from build123d import *

# Parameters (mm, degrees)
F2_DEPTH = 5
F1_W     = 60
F1_H     = 60
F3_DEPTH = 2


# Not quite as in the source:
# - ends of sketch curves that miss each other by under 0.0002 mm in the source are joined


with BuildPart() as f2:
    # F0 (on Top) → F2 (new body)
    with BuildSketch(Plane.XY):
        with BuildLine():
            Line((12.5301, 15.3483), (13.2754, 18.8292))
            ThreePointArc((13.2754, 18.8292), (-0.0620714554, 21.313337159), (-13.4587020592, 19.1710971727))
            Line((-13.4587020592, 19.1710971727), (-12.8601, 15.6049))
            Line((-12.8601, 15.6049), (-0.5682, 9.3636))
            Line((-0.5682, 9.3636), (12.5301, 15.3483))
        make_face()
        Polygon((5.0768, 17.1559), (-0.2261, 13.5284), (-5.468, 17.1559), align=None, mode=Mode.SUBTRACT)
    extrude(amount=F2_DEPTH)



with BuildPart() as f2b:
    # F0 (on Top) → F2, piece 2 (new body)
    with BuildSketch(Plane.XY):
        Polygon((20.3255, 19.4397), (14.8884, 19.4397), (13.6053, 14.2734), (4.869, 10.0354), (3.3296, 1.7791), (12.2, 1.7791), (17.6374, 5.1989), align=None)
        Polygon((15.3523, 8.6188), (15.3523, 7.3484), (5.7369, 3.3912), (5.7369, 4.9303), align=None, mode=Mode.SUBTRACT)
        Polygon((16.3548, 12.6613), (16.3548, 11.2445), (6.9587, 7.5562), (6.9587, 8.9606), align=None, mode=Mode.SUBTRACT)
    extrude(amount=F2_DEPTH)


with BuildPart() as f2c:
    # F0 (on Top) → F2, piece 3 (new body)
    with BuildSketch(Plane.XY):
        Polygon((-4.0627, 1.9012), (-5.6145, 10.2308), (-13.9352, 14.5301), (-15.0105, 19.9041), (-20.3255, 19.9041), (-17.8452, 5.7363), (-12.3223, 1.9012), align=None)
        Polygon((-16.098, 9.4248), (-6.3597, 5.3332), (-6.3597, 3.9288), (-15.9514, 8.1913), align=None, mode=Mode.SUBTRACT)
        Polygon((-16.6601, 13.6628), (-7.2887, 9.4248), (-7.2152, 7.947), (-16.5379, 12.1483), align=None, mode=Mode.SUBTRACT)
    extrude(amount=F2_DEPTH)


with BuildPart() as f2d:
    # F0 (on Top) → F2, piece 4 (new body)
    with BuildSketch(Plane.XY):
        Polygon((-14.0697, -1.5185), (-14.4852, 1.7669), (-17.5644, 3.7209), (-16.3667, -15.1486), (-9.0357, -18.9712), (-8.9623, -4.7428), align=None)
    extrude(amount=F2_DEPTH)


with BuildPart() as f2e:
    # F0 (on Top) → F2, piece 5 (new body)
    with BuildSketch(Plane.XY):
        Polygon((17.161, 3.318), (13.6663, 0.8999), (13.5321, -1.6531), (8.0952, -4.938), (8.0952, -19.2404), (15.6947, -15.8937), align=None)
    extrude(amount=F2_DEPTH)


with BuildPart() as f2f:
    # F0 (on Top) → F2, piece 6 (new body)
    with BuildSketch(Plane.XY):
        Polygon((-3.794, 9.2295), (-2.6575, 2.3167), (-2.6575, -10.5809), (1.8513, -10.5809), (1.8513, 2.4509), (3.1219, 9.2295), (-0.5682, 7.6783), align=None)
    extrude(amount=F2_DEPTH)


with BuildPart() as f2g:
    # F0 (on Top) → F2, piece 7 (new body)
    with BuildSketch(Plane.XY):
        Polygon((-7.4959, -4.7428), (-7.4959, -19.4476), (-6.0788, -20.4494), (-4.1971, -14.2084), (3.1219, -14.2084), (5.0647, -20.3757), (6.6777, -19.5086), (6.6777, -4.7428), (3.3906, -1.7137), (3.3906, -11.8511), (-4.0627, -11.8511), (-4.1971, -1.7137), align=None)
    extrude(amount=F2_DEPTH)


with BuildPart() as f2h:
    # F0 (on Top) → F2, piece 8 (new body)
    with BuildSketch(Plane.XY):
        Polygon((-3.2564, -15.5518), (-4.7349, -21.3286), (3.7325, -21.3286), (2.047, -15.5518), align=None)
    extrude(amount=F2_DEPTH)


with BuildPart() as f2_1:
    add(f2.part)

    add(f2b.part)  # F3 merges F2b

    add(f2c.part)  # F3 merges F2c

    add(f2d.part)  # F3 merges F2d

    add(f2e.part)  # F3 merges F2e

    add(f2f.part)  # F3 merges F2f

    add(f2g.part)  # F3 merges F2g

    add(f2h.part)  # F3 merges F2h
    # F1 (on Top) → F3 (join)
    with BuildSketch(Plane.XY):
        Rectangle(F1_W, F1_H)
    extrude(amount=F3_DEPTH)


solid = f2_1.part
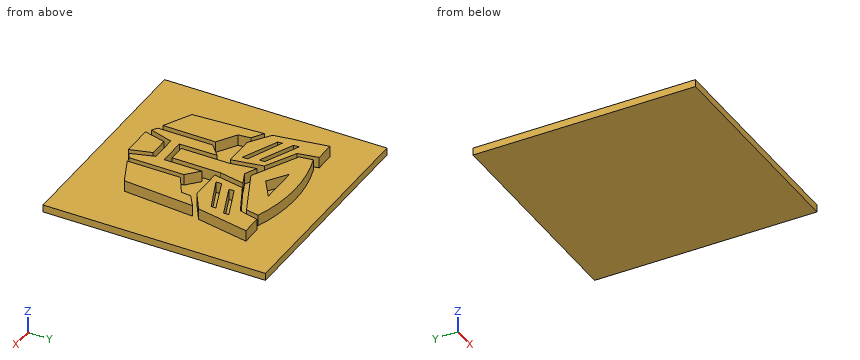
The listing builds one solid part. Answer for the finished solid, in the listing's coordinates (mm). Coordinates: 2 decimals unless noted, no trailing zeros. Loops run counter-clockwise (first coordinate to the right, second up) from the corner with the lowest first, then second, coordinate; pieces in that order, holes last. Notation, with made-up numbers: (26.25, 48) -> (41.25, 48) arc R18 ccw to (41.25, 62) -> close; hole circle Ø11 at (7, 37.25). An arc over 180 degrees is marked (long way). Answer in a Markdown table with one row per item. Add a question column.
1. The part is cut by section B-B, the plane y = 0. Write down the section's boundary in (x, z), then the cut area to 3 significant figures.
2. The part is cut by section A-A, the plane z = 3.85. Count the separate pieces of the cut face and the enclosed holes in it, then the cut area to 3 significant figures.
3. The part is cut by section D-D, the plane x = -23. Write down the section's boundary in (y, z).
4. Flat-ended cylindrical pins translate along their axes: P1, Ø1.5, axis at x = -8, z = 3.5, coming from the -Y side; P2, Ø2.5, axis at x = -2.5, z = 4, coming from the -Y side; P3, Ø2.5, axis at y = -2, z = 3.5, coming from the -X side. Find the tip coordinate at first contact, or state that the pin passes through.
5. Consider line 1 (X direction, y = 4, z = 3.75); line 2 (X direction, y = 15.5, z = 4.4); line 3 (Z direction, x = -21, y = 5.5). Determine where each line is inside the solid, lowest interval first. Write a range as [from, to].
6. The part is cut by section C-C, the plane x = 9.5. Write down the section's boundary in (y, z).
Answer below:
| question | item | result |
|---|---|---|
| 1 | outline | (-30, 0) -> (30, 0) -> (30, 2) -> (16.91, 2) -> (16.91, 5) -> (13.62, 5) -> (13.62, 2) -> (1.85, 2) -> (1.85, 5) -> (-2.66, 5) -> (-2.66, 2) -> (-14.26, 2) -> (-14.26, 5) -> (-17.33, 5) -> (-17.33, 2) -> (-30, 2) -> close |
| 1 | area | 153 mm2 |
| 2 | separate pieces | 8 |
| 2 | enclosed holes | 5 |
| 2 | area | 991 mm2 |
| 3 | outline | (-30, 0) -> (30, 0) -> (30, 2) -> (-30, 2) -> close |
| 4 | P1 | y = -19.62 |
| 4 | P2 | y = -21.33 |
| 4 | P3 | x = -17.28 |
| 5 | line 1 | [-15.34, -6.52], [-6.36, -4.45], [-2.93, 2.14], [3.74, 5.74], [7.22, 15.73] |
| 5 | line 2 | [-19.55, -14.13], [-12.65, -3.08], [2.66, 12.56], [13.91, 19.58] |
| 5 | line 3 | [0, 2] |
| 6 | outline | (-30, 0) -> (30, 0) -> (30, 2) -> (20.02, 2) -> (20.02, 5) -> (13.96, 5) -> (13.96, 2) -> (12.28, 2) -> (12.28, 5) -> (9.96, 5) -> (9.96, 2) -> (8.55, 2) -> (8.55, 5) -> (6.37, 5) -> (6.37, 2) -> (4.94, 2) -> (4.94, 5) -> (1.78, 5) -> (1.78, 2) -> (-4.09, 2) -> (-4.09, 5) -> (-18.62, 5) -> (-18.62, 2) -> (-30, 2) -> close |
